```python
from build123d import *

# Parameters (mm, degrees)
SKETCH1_R           = 95
BOSS_EXTRUDE1_DEPTH = 500
SHELL1_T            = 10
SKETCH2_R           = 30
BOSS_EXTRUDE2_DEPTH = 20
SKETCH4_R           = 20
BOSS_EXTRUDE3_DEPTH = 95


with BuildPart() as part:
    # Sketch1 → Boss-Extrude1 (new body)
    with BuildSketch(Plane(origin=(0, 0, 0), x_dir=(1, 0, 0), z_dir=(0, 1, 0))):
        Circle(SKETCH1_R)
    extrude(amount=BOSS_EXTRUDE1_DEPTH)

    # Shell1 (no face opened: a closed hollow body)
    add(offset(amount=-SHELL1_T, mode=Mode.PRIVATE), mode=Mode.SUBTRACT)

    # Sketch2 → Boss-Extrude2 (add)
    with BuildSketch(Plane(origin=(0, 0, -95), x_dir=(-1, 0, 0), z_dir=(0, 0, -1))):
        with BuildLine():
            Line((0, 0), (95, 0))
            Line((95, 0), (217.806884991, 32.302770759))
            ThreePointArc((217.806884991, 32.302770759), (270, 100), (217.806884991, 167.697229241))
            Line((217.806884991, 167.697229241), (95, 200))
            Line((95, 200), (0, 200))
            Line((0, 200), (0, 0))
        make_face()
        with Locations((200, 100)):
            Circle(SKETCH2_R, mode=Mode.SUBTRACT)
        with BuildLine():
            Line((0, 500), (95, 500))
            Line((95, 500), (179.519741664, 452.235857915))
            ThreePointArc((179.519741664, 452.235857915), (210, 400), (179.519741664, 347.764142085))
            Line((179.519741664, 347.764142085), (95, 300))
            Line((95, 300), (0, 300))
            Line((0, 300), (0, 500))
        make_face()
    boss_extrude2 = extrude(amount=-BOSS_EXTRUDE2_DEPTH)

    # Mirror1: Boss-Extrude2 across plane
    add(boss_extrude2.mirror(Plane(origin=(0, 0, 0), x_dir=(1, 0, 0), z_dir=(0, 0, -1))))

    # Sketch4 → Boss-Extrude3 (add, symmetric)
    with BuildSketch(Plane.XY):
        with Locations((-150, 400)):
            Circle(SKETCH4_R)
    extrude(amount=BOSS_EXTRUDE3_DEPTH, both=True)


solid = part.part
```
Source: CAD feature listing. Evaluate the final solid. Frame: model axes, mm. A direction names the side the tool comes from. Round coordinates to 2 decimals unless told otherwise and drop trailing zeros. Write each loop counter-clockwise with the first axis right and the second up, starting at its lowest first coordinate (ties: lowest second). Pieces come first, ordered by that corner, then holes. Notation, with made-up numbers: M 22,-10 L 58,-10 A22 ccw 58,23 Z; hole C 56.25,47.25 d3. An arc over 180 degrees is marked long. Answer as a JSON object with one key per item and string values. Group by question number.
(1) Reachability of faces 5 (the flat face through (-69, 200, 87)), 6 (the flat face through (-20, 106, 75)), 7 (the flat face through (-1, 500, -1)), 8 (the flat face through (-137.852, 324.216, 85.14)) from +Z, -Z, +X, -X, +Y, -Y: full face, straight path, thin tool, end or side. Return the list, or none.
(2) First-contact query: pin 1 (10 mm diameter, centred on x = -143, z = 68, fed in from -Y); pin 2 (6 mm diameter, centred on x = -41.5, z = -82, fed in from -Y); pin 3 (6 mm diameter, centred on x = 47.5, y = 397.5, fed in from +Z); pin 4 (10 mm diameter, centred on x = -166, z = -33.5, fed in from -Y). Flat tips, straight axial feed; report the tip coordinate or a pass-through.
(3) Section query C-C on y = 400. Output: boundary loops of the cut face in (x, z), then the cut area to 3 significant figures.
(4) Section query B-B on x = -200. Output: boundary loops of the cut face in (y, z), then the cut area to 3 significant figures.
(5) Section query A-A on z = 0. Output: boundary loops of the cut face in (x, y).
(6) Section query D-D on z = 24. Output: boundary loops of the cut face in (x, y), then the cut area to 3 significant figures.
(7) Mould query, pull axis X, two halves, no side actions, for faces 1 (the flat face through (-69, 200, -87)), 2 (the flat face through (-20, 106, -75)), 3 (the flat face through (-136.67, 476.45, -85.14)), 4 (the flat face through (-1, 10, -1)). Classes: +X half, -X half, draft (parallel to the pull), parting line (faces both ways), or undercut.
(8) Ray query, line 1 (Y direction, x = -53.5, z = 55.5); line 2 (Y direction, x = -200, z = 82); line 3 (Z direction, x = -122, y = 149). Return the intervals inside material, ascending. Write a range as [from, to].
Computed values:
{
 "1": {"face 5": "+Z, -X", "face 6": "none", "face 7": "+Z, -Z, +X, -X, +Y", "face 8": "+Z, -Z, -X"},
 "2": {"pin 1": "y = 380.1", "pin 2": "y = 0", "pin 3": "z = 83.93", "pin 4": "y = 383.3"},
 "3": {"outline": "M -210,-95 L 0,-95 A95 ccw 0,95 L -210,95 L -210,75 L -170,75 L -170,-75 L -210,-75 Z; hole M -130,-75 L -58.31,-75 A95 cw -58.31,75 L -130,75 Z; hole M -40,-75 L 0,-75 L 0,-85 A85 ccw 0,85 L 0,75 L -40,75 A85 ccw Z", "area": "19,000 mm^2"},
 "4": {"outline": "M 27.62,-95 L 70,-95 L 70,-75 L 27.62,-75 Z; M 27.62,75 L 70,75 L 70,95 L 27.62,95 Z; M 130,-95 L 172.38,-95 L 172.38,-75 L 130,-75 Z; M 130,75 L 172.38,75 L 172.38,95 L 130,95 Z; M 366.83,-95 L 433.17,-95 L 433.17,-75 L 366.83,-75 Z; M 366.83,75 L 433.17,75 L 433.17,95 L 366.83,95 Z", "area": "6,040 mm^2"},
 "5": {"outline": "C -150,400 d40; M -95,0 L 95,0 L 95,500 L -95,500 Z; hole M -85,10 L 85,10 L 85,490 L -85,490 Z"},
 "6": {"outline": "C -150,400 d40; M -91.92,0 L 91.92,0 L 91.92,500 L -91.92,500 Z; hole M -81.54,10 L 81.54,10 L 81.54,490 L -81.54,490 Z", "area": "14,900 mm^2"},
 "7": {"face 1": "draft", "face 2": "undercut", "face 3": "-X half", "face 4": "undercut"},
 "8": {"line 1": "[0, 10], [490, 500]", "line 2": "[27.62, 70], [130, 172.38], [366.83, 433.17]", "line 3": "[-95, -75], [75, 95]"}
}
